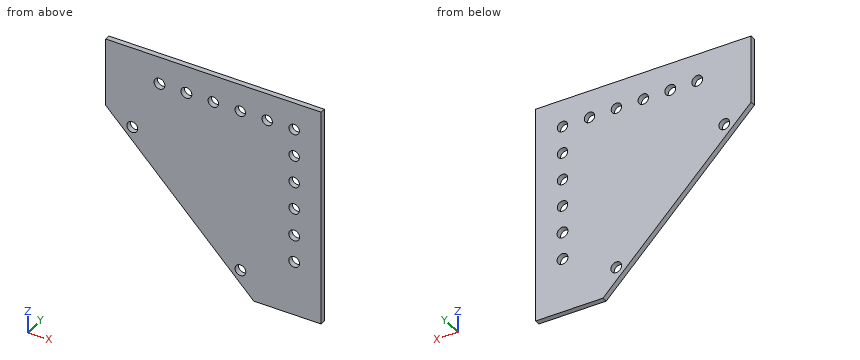
```python
from build123d import *

# Parameters (mm, degrees)
BOSS_EXTRUDE1_DEPTH          = 1.27
F_10_0_1935_DIAMETER_HOLE1_D = 4.9149
F_10_CLEARANCE_HOLE3_D       = 5.1054
SKETCH8_W                    = 182.273007985
SKETCH8_H                    = 142.759278982
SKETCH8_W_2                  = 101.6
SKETCH8_H_2                  = 101.6
CUT_EXTRUDE1_DEPTH           = 114.076021494


with BuildPart() as part:
    # Sketch1 → Boss-Extrude1 (new, symmetric)
    with BuildSketch(Plane(origin=(0, 0, 0), x_dir=(1, 0, 0), z_dir=(0, 1, 0))):
        with BuildLine():
            Line((53.835856574, 81.994245871), (53.835856574, -36.025498008))
            Line((53.835856574, -36.025498008), (-64.183887305, -36.025498008))
            ThreePointArc((-64.183887305, -36.025498008), (-70.050522337, -32.105537803), (-68.674015366, -25.185369947))
            Line((-68.674015366, -25.185369947), (42.995728513, 86.484373931))
            ThreePointArc((42.995728513, 86.484373931), (49.915896369, 87.860880902), (53.835856574, 81.994245871))
        make_face()
    extrude(amount=BOSS_EXTRUDE1_DEPTH, both=True)

    # #10 (0.1935) Diameter Hole1 (through all)
    with Locations(Plane(origin=(0, 1.27, 0), x_dir=(1, 0, 0), z_dir=(0, 1, 0))):
        with Locations((41.135856574, -23.325498008), (28.435856574, -23.325498008), (15.735856574, -23.325498008), (3.035856574, -23.325498008), (41.135856574, -10.625498008), (41.135856574, 2.074501992), (41.135856574, 14.774501992)):
            Hole(F_10_0_1935_DIAMETER_HOLE1_D / 2)

    # #10 Clearance Hole3 (through all)
    with Locations(Plane(origin=(0, 1.27, 0), x_dir=(1, 0, 0), z_dir=(0, 1, 0))):
        with Locations((-9.664143426, -23.325498008), (-22.364143426, -23.325498008), (41.135856574, 27.474501992), (41.135856574, 40.174501992), (15.795798418, 52.929822822), (-35.153913001, 1.902635256)):
            Hole(F_10_CLEARANCE_HOLE3_D / 2)

    # Sketch8 → Cut-Extrude1 (cut, through all)
    with BuildSketch(Plane(origin=(0, 1.27, 0), x_dir=(1, 0, 0), z_dir=(0, 1, 0))):
        with Locations((14.049390588, 20.35997908)):
            Rectangle(SKETCH8_W, SKETCH8_H)
        with Locations((3.035856574, 14.774501992)):
            Rectangle(SKETCH8_W_2, SKETCH8_H_2, mode=Mode.SUBTRACT)
    extrude(amount=-CUT_EXTRUDE1_DEPTH, mode=Mode.SUBTRACT)


solid = part.part
```
Geometry: final body of the model. Coordinates: model frame, mm. Coordinates: 2 decimals unless noted, no trailing zeros. Loops run counter-clockwise (first coordinate to the right, second up) from the corner with the lowest first, then second, coordinate; pieces in that order, holes last. Notation, with made-up numbers: (48.25, 0.5) -> (62.25, 0.5) arc R19 ccw to (62.25, 13.5) -> close; hole circle Ø9 at (53, 12). An arc over 180 degrees is marked (long way). Use a Markdown table: item, result. Add a question column.
(1) Section query A-A, the plane x = 17. Return loops of the section in (y, z), plus the area to 3 significant figures.
(2) Line query: line 1 along Z through (x, y) = (16, -1.1); line 2 along X through (y, z) = (-0.15, 12); line 3 along X through (y, z) = (0.25, -29). Output: solid intervals per line, ascending.
(3) Section query D-D, the plane z = -32. Return loops of the section in (x, y), plus the area to 3 significant figures.
(4) Section query C-C, the plane x = -22. Return loops of the section in (y, z), plus the area to 3 significant figures.
(5) Section query B-B, the plane y = -0.7. State how many separate pieces and enclosed holes the cut face has, plus the area to 3 significant figures.
(6) Pin query (flat end, axial travel): pin 1 Ø4 at (x, z) = (-35.15, -1.9) entering from +Y. Return the tip coordinate at first contact, or that it passes through.
Answer:
| question | item | result |
|---|---|---|
| 1 | outline | (-1.27, -60.49) -> (1.27, -60.49) -> (1.27, -55.18) -> (-1.27, -55.18) -> close; (-1.27, -50.68) -> (1.27, -50.68) -> (1.27, 21.22) -> (-1.27, 21.22) -> close; (-1.27, 25.43) -> (1.27, 25.43) -> (1.27, 36.03) -> (-1.27, 36.03) -> close |
| 1 | area | 223 mm^2 |
| 2 | line 1 | z = -59.49 to -55.47, -50.39 to 20.88, 25.77 to 36.03 |
| 2 | line 2 | x = -47.76 to 39.1, 43.17 to 53.84 |
| 2 | line 3 | x = -14.49 to 39.09, 43.18 to 53.84 |
| 3 | outline | (-11.49, -1.27) -> (53.84, -1.27) -> (53.84, 1.27) -> (-11.49, 1.27) -> close |
| 3 | area | 166 mm^2 |
| 4 | outline | (-1.27, -21.49) -> (1.27, -21.49) -> (1.27, 20.8) -> (-1.27, 20.8) -> close; (-1.27, 25.85) -> (1.27, 25.85) -> (1.27, 36.03) -> (-1.27, 36.03) -> close |
| 4 | area | 133 mm^2 |
| 5 | separate pieces | 1 |
| 5 | enclosed holes | 13 |
| 5 | area | 7,630 mm^2 |
| 6 | pin 1 | passes through |
